```python
from build123d import *

# Parameters (mm, degrees)
F1_DEPTH = 7.14375
F2_R     = 2.4511
F3_DEPTH = 7.14475
F4_R     = 3.3655
F5_DEPTH = 5.9436


with BuildPart() as f1:
    # F0 (on Front) → F1 (new body)
    with BuildSketch(Plane.XZ):
        Polygon((-2.644188, 4.653896), (-5.352486, 0.037014), (-2.708298, -4.616882), (2.644188, -4.653896), (5.352486, -0.037014), (2.708298, 4.616882), align=None)
    extrude(amount=F1_DEPTH)

    # F2 (on face) → F3 (cut, through all)
    with BuildSketch(Plane.XZ.offset(7.14375)):
        Circle(F2_R)
    extrude(amount=-F3_DEPTH, mode=Mode.SUBTRACT)

    # F4 (on face) → F5 (cut)
    with BuildSketch(Plane.XZ.offset(7.14375)):
        Circle(F4_R)
    extrude(amount=-F5_DEPTH, mode=Mode.SUBTRACT)


solid = f1.part
```
Build history of the part. All positions in model axes, mm. A direction names the side the tool comes from. Round coordinates to 2 decimals unless told otherwise and drop trailing zeros. Order: outer loops, then holes, each group sorted by start corner. A loop starts at its lowest first (then second) coordinate and runs counter-clockwise, first axis right, second up. Notation, with made-up numbers: (30.5, 87) -> (70.5, 87) arc R27 cw to (70.5, 109) -> close; hole circle Ø4 at (81.5, -10.75). An arc over 180 degrees is marked (long way). Answer in a Markdown table with one row per item.
1) Pin check, flat tips, straight feed: P1, Ø2, axis at x = -4, y = -6, coming from the -Z side; P2, Ø1, axis at x = 0, y = -1, coming from the +Z side. Stop position of each tip, or through.
Values:
| item | result |
|---|---|
| P1 | z = -4.1 |
| P2 | z = 4.64 |
2) Band-saw the part on B-B on z = -2.25. Give the cut face in (x, y).
Values:
| item | result |
|---|---|
| outline | (-4.05, -7.14) -> (-2.5, -7.14) -> (-2.5, -1.2) -> (-0.97, -1.2) -> (-0.97, 0) -> (-4.05, 0) -> close; (0.97, -1.2) -> (2.5, -1.2) -> (2.5, -7.14) -> (4.05, -7.14) -> (4.05, 0) -> (0.97, 0) -> close |
3) Mould opens along Z. For faces 3 (the flat face through (4.049, -3.522, 2.257)), 4 (the flat face through (-2, -1.2, -2)), 5 (the flat face through (-4.049, -3.522, -2.257)), 6 (the flat face through (3.5, -7.144, 1.1)) say: released by +Z, released by -Z, zero draft, split by the parting line, or undercut.
Values:
| item | result |
|---|---|
| face 3 | released by +Z |
| face 4 | undercut |
| face 5 | released by -Z |
| face 6 | zero draft |
4) Band-saw the part on C-C on x = 2. Give the cut face in (y, z).
Values:
| item | result |
|---|---|
| outline | (-7.14, -4.65) -> (0, -4.65) -> (0, -1.42) -> (-1.2, -1.42) -> (-1.2, -2.71) -> (-7.14, -2.71) -> close; (-7.14, 2.71) -> (-1.2, 2.71) -> (-1.2, 1.42) -> (0, 1.42) -> (0, 4.62) -> (-7.14, 4.62) -> close |
5) Which spindle directions (+Z, -Z, +X, -X, +Y, -Y) get a long thin tool onto all of the face, cutting with end or side? Do faces 1 (the cylindrical face through (-2.67, -4.21, -2.05)), 2 (the flat face through (-2.5, 0, 1.1)). Say none if no direction does.
Values:
| item | result |
|---|---|
| face 1 | -Y |
| face 2 | +Z, -Z, +X, -X, +Y |
6) Band-saw the part on D-D on z = 3. Give the cut face in (x, y).
Values:
| item | result |
|---|---|
| outline | (-3.61, -7.14) -> (-1.53, -7.14) -> (-1.53, -1.2) -> (1.53, -1.2) -> (1.53, -7.14) -> (3.63, -7.14) -> (3.63, 0) -> (-3.61, 0) -> close |
7) Wall check: L1, parallel to Y at x = 0, z = -2.5; L2, parallel to Z at x = 0, y = -3.5; L3, parallel to X at y = -2, z = 1.5. Give the ranges that are in metal, low to high.
Values:
| item | result |
|---|---|
| L1 | -1.2 to 0 |
| L2 | -4.64 to -3.37, 3.37 to 4.64 |
| L3 | -4.49 to -3.01, 3.01 to 4.48 |
8) Band-saw the part on A-A on y = -3. Give the cut face in (x, z).
Values:
| item | result |
|---|---|
| outline | (-5.35, 0.04) -> (-2.71, -4.62) -> (2.64, -4.65) -> (5.35, -0.04) -> (2.71, 4.62) -> (-2.64, 4.65) -> close; hole circle Ø6.73 at (0, 0) |
